from build123d import *

# Parameters (mm, degrees)
SKETCH1_W            = 152.4
SKETCH1_H            = 101.6
EXTRUDE1_DEPTH       = 25.4
SKETCH2_R            = 6.35
CUT_EXTRUDE2_DEPTH   = 96.038097624
LPATTERN1_COUNT      = 2
LPATTERN1_PITCH      = 50.8
LPATTERN1_COUNT_DIR2 = 2
LPATTERN1_PITCH_DIR2 = 50.8
SKETCH3_R            = 12.7
CUT_EXTRUDE3_DEPTH   = 96.038097624
LPATTERN2_COUNT      = 2
LPATTERN2_PITCH      = 63.5
LPATTERN2_COUNT_DIR2 = 2
LPATTERN2_PITCH_DIR2 = 114.3
CHAMFER1_SIZE        = 1.524
SKETCH4_R            = 17.4625
CUT_EXTRUDE5_DEPTH   = 96.038097624
LPATTERN3_COUNT      = 3
LPATTERN3_PITCH      = 41.275


with BuildPart() as part:
    # Sketch1 → Extrude1 (new body)
    with BuildSketch(Plane.XY):
        Rectangle(SKETCH1_W, SKETCH1_H)
    extrude(amount=-EXTRUDE1_DEPTH)

    # Sketch2 → Cut-Extrude2 (cut, through all)
    with BuildSketch(Plane(origin=(0, 0, -25.4), x_dir=(1, 0, 0), z_dir=(0, 0, -1))):
        with Locations(Location((-25.4, -25.4, 0), (0, 0, 270))):
            Circle(SKETCH2_R)
    cut_extrude2 = extrude(amount=-CUT_EXTRUDE2_DEPTH, mode=Mode.SUBTRACT)

    # LPattern1: Cut-Extrude2 2 × 2
    with Locations(*[(i * LPATTERN1_PITCH, -j * LPATTERN1_PITCH_DIR2, 0) for i in range(LPATTERN1_COUNT) for j in range(LPATTERN1_COUNT_DIR2) if (i, j) != (0, 0)]):
        add(cut_extrude2, mode=Mode.SUBTRACT)

    # Sketch3 → Cut-Extrude3 (cut, through all)
    with BuildSketch(Plane(origin=(0, 0, -25.4), x_dir=(1, 0, 0), z_dir=(0, 0, -1))):
        with Locations(Location((57.15, 31.75, 0), (0, 0, 270))):
            Circle(SKETCH3_R)
    cut_extrude3 = extrude(amount=-CUT_EXTRUDE3_DEPTH, mode=Mode.SUBTRACT)

    # LPattern2: Cut-Extrude3 2 × 2
    with Locations(*[(-j * LPATTERN2_PITCH_DIR2, i * LPATTERN2_PITCH, 0) for i in range(LPATTERN2_COUNT) for j in range(LPATTERN2_COUNT_DIR2) if (i, j) != (0, 0)]):
        add(cut_extrude3, mode=Mode.SUBTRACT)

    # Chamfer1
    chamfer1_edges = [part.edges().sort_by_distance(p)[0] for p in [
        (76.2, 0, -25.4),
        (0, 50.8, -25.4),
        (-76.2, 0, -25.4),
        (0, 50.8, 0),
        (76.2, 0, 0),
        (0, -50.8, 0),
        (-76.2, 0, 0),
        (0, -50.8, -25.4),
        (-76.2, 50.8, -12.7),
        (76.2, 50.8, -12.7),
        (76.2, -50.8, -12.7),
        (-76.2, -50.8, -12.7),
    ]]
    chamfer(chamfer1_edges, length=CHAMFER1_SIZE)

    # Sketch4 → Cut-Extrude5 (cut, through all)
    with BuildSketch(Plane.XY):
        with Locations((41.275, 0)):
            Circle(SKETCH4_R)
    cut_extrude5 = extrude(amount=-CUT_EXTRUDE5_DEPTH, mode=Mode.SUBTRACT)

    # LPattern3: Cut-Extrude5 ×3
    with Locations(*[(-i * LPATTERN3_PITCH, 0, 0) for i in range(1, LPATTERN3_COUNT)]):
        add(cut_extrude5, mode=Mode.SUBTRACT)


solid = part.part
For this review, take the finished solid that the model builds, in its own axes (mm). Coordinates: 2 decimals unless noted, no trailing zeros. Write each loop counter-clockwise with the first axis right and the second up, starting at its lowest first coordinate (ties: lowest second). Pieces come first, ordered by that corner, then holes. Notation, with made-up numbers: (-9, 11.25) -> (16, 11.25) arc R10 cw to (16, 24.25) -> close; hole circle Ø10 at (-20, 10.25). An arc over 180 degrees is marked (long way). Write each question's results on one line, items separated by ' | '. Start each with the question number.
1) Wall thickness on L1, parallel to Y at x = -22.5, z = -18.75; L2, parallel to X at y = 33, z = -16; L3, parallel to X at y = 16, z = -12.5: over which ranges is each line inside the solid? List them lowest first. Write a range as [from, to].
2) Consider section C-C (x = -49). Write out the cut boundary in (y, z).
3) Consider section B-B (z = -7). Give the number of separate pieces and of enclosed holes in the cut face, plus the area to 3 significant figures.
4) The part is to be moulded in two halves that separate along Y. For faces 1 (the face through (-76.2, -1, -13)), 2 (the face through (-31.034, -22.47, -12.878)), 3 (the face through (-1, -50.8, -13)), say which applies: +Y half, -Y half, draft (parallel to the pull), parting line (faces both ways), or undercut.
5) Insertion check: pin 1 (15 mm diameter, centred on x = 57.15, y = 31.75, fed in from +Z). The pin has a flat end and moves straight along its axis. Give the tip position at first contact, or say it passes through.
6) Consider section D-D (y = -29.5). Write out the cut boundary in (x, z).
7) Consider section A-A (y = 3). Write out the cut boundary in (x, z), plus the area to 3 significant figures.
Geometry says:
1) L1: [-50.8, -31.05], [-19.75, 19.75], [31.05, 50.8] | L2: [-76.2, -69.79], [-44.51, 44.51], [69.79, 76.2] | L3: [-76.2, -48.27], [-34.28, -7], [7, 34.28], [48.27, 76.2]
2) outline: (-50.8, -23.88) -> (-49.28, -25.4) -> (-41.49, -25.4) -> (-41.49, 0) -> (-49.28, 0) -> (-50.8, -1.52) -> close; (-22.01, -25.4) -> (-15.66, -25.4) -> (-15.66, 0) -> (-22.01, 0) -> close; (15.66, -25.4) -> (22.01, -25.4) -> (22.01, 0) -> (15.66, 0) -> close; (41.49, -25.4) -> (49.28, -25.4) -> (50.8, -23.88) -> (50.8, -1.52) -> (49.28, 0) -> (41.49, 0) -> close
3) separate pieces: 1 | enclosed holes: 11 | area: 10,100 mm^2
4) face 1: draft | face 2: undercut | face 3: -Y half
5) pin 1: through
6) outline: (-76.2, -23.88) -> (-74.68, -25.4) -> (-69.65, -25.4) -> (-69.65, 0) -> (-74.68, 0) -> (-76.2, -1.52) -> close; (-44.65, -25.4) -> (-30.25, -25.4) -> (-30.25, 0) -> (-44.65, 0) -> close; (-20.55, -25.4) -> (20.55, -25.4) -> (20.55, 0) -> (-20.55, 0) -> close; (30.25, -25.4) -> (44.65, -25.4) -> (44.65, 0) -> (30.25, 0) -> close; (69.65, -25.4) -> (74.68, -25.4) -> (76.2, -23.88) -> (76.2, -1.52) -> (74.68, 0) -> (69.65, 0) -> close
7) outline: (-76.2, -23.88) -> (-74.68, -25.4) -> (-58.48, -25.4) -> (-58.48, 0) -> (-74.68, 0) -> (-76.2, -1.52) -> close; (-24.07, -25.4) -> (-17.2, -25.4) -> (-17.2, 0) -> (-24.07, 0) -> close; (17.2, -25.4) -> (24.07, -25.4) -> (24.07, 0) -> (17.2, 0) -> close; (58.48, -25.4) -> (74.68, -25.4) -> (76.2, -23.88) -> (76.2, -1.52) -> (74.68, 0) -> (58.48, 0) -> close | area: 1,240 mm^2
